Geometry check sheet. Reference: the model listing, model coordinates, mm. Coordinates: 2 decimals unless noted, no trailing zeros. Order: outer loops, then holes, each group sorted by start corner. A loop starts at its lowest first (then second) coordinate and runs counter-clockwise, first axis right, second up. Notation, with made-up numbers: (-34.5, -19) -> (6.5, -19) arc R11 cw to (6.5, -6) -> close; hole circle Ø5 at (42, -21). An arc over 180 degrees is marked (long way). Answer in a Markdown table with one row per item. Add a question column.
```python
from build123d import *

# Parameters (mm, degrees)
SKETCH_1_W          = 30
SKETCH_1_H          = 26.5
EXTRUDE_1_DEPTH     = 3
SKETCH_2_R          = 5
CUT_EXTRUDE_1_DEPTH = 30.15187029
SKETCH_3_R          = 2
CUT_EXTRUDE_2_DEPTH = 30.15187029
EXTRUDE_3_DEPTH     = 3
SKETCH_7_R          = 4
SKETCH_7_R_2        = 1.6
CUT_EXTRUDE_3_DEPTH = 3
FILLET_1_R          = 2
FILLET_2_R          = 2


with BuildPart() as part:
    # 草图1 → 凸台-拉伸1 (new body)
    with BuildSketch(Plane(origin=(0, 0, 0), x_dir=(1, 0, 0), z_dir=(0, 1, 0))):
        with Locations((-10.540723982, -0.479638009)):
            Rectangle(SKETCH_1_W, SKETCH_1_H)
    extrude(amount=EXTRUDE_1_DEPTH)

    # 草图2 → 切除-拉伸1 (cut, through all)
    with BuildSketch(Plane(origin=(0, 3, 0), x_dir=(1, 0, 0), z_dir=(0, 1, 0))):
        with Locations(Location((-10.540723982, -0.479638009, 0), (0, 0, 270))):
            Circle(SKETCH_2_R)
    extrude(amount=-CUT_EXTRUDE_1_DEPTH, mode=Mode.SUBTRACT)

    # 草图3 → 切除-拉伸2 (cut, through all)
    with BuildSketch(Plane(origin=(0, 3, 0), x_dir=(1, 0, 0), z_dir=(0, 1, 0))):
        with Locations(Location((-3.540723982, 7.520361991, 0), (0, 0, 270))):
            Circle(SKETCH_3_R)
        with Locations(Location((-17.540723982, 7.520361991, 0), (0, 0, 270))):
            Circle(SKETCH_3_R)
        with Locations(Location((-3.540723982, -8.479638009, 0), (0, 0, 270))):
            Circle(SKETCH_3_R)
        with Locations(Location((-17.540723982, -8.479638009, 0), (0, 0, 270))):
            Circle(SKETCH_3_R)
    extrude(amount=-CUT_EXTRUDE_2_DEPTH, mode=Mode.SUBTRACT)

    # 草图6 → 凸台-拉伸3 (add)
    with BuildSketch(Plane(origin=(4.459276018, 0, 0), x_dir=(0, 0, -1), z_dir=(1, 0, 0))):
        with BuildLine():
            Line((12.770361991, 3), (-13.729638009, 3))
            Line((-13.729638009, 3), (-13.729638009, -16.75))
            ThreePointArc((-13.729638009, -16.75), (-0.479638009, -30), (12.770361991, -16.75))
            Line((12.770361991, -16.75), (12.770361991, 3))
        make_face()
    extrude(amount=EXTRUDE_3_DEPTH)

    # 草图7 → 切除-拉伸3 (cut)
    with BuildSketch(Plane.ZY.offset(-4.459276018)):
        with Locations((0.479638009, -16.75)):
            Circle(SKETCH_7_R)
        with Locations((9.432771386, -16.75)):
            Circle(SKETCH_7_R_2)
        with Locations((-7.567228614, -16.75)):
            Circle(SKETCH_7_R_2)
    extrude(amount=-CUT_EXTRUDE_3_DEPTH, mode=Mode.SUBTRACT)

    # 圆角1
    fillet_1_edges = [part.edges().sort_by_distance(p)[0] for p in [
        (-25.540723982, 1.5, -12.770361991),
        (-25.540723982, 1.5, 13.729638009),
    ]]
    fillet(fillet_1_edges, radius=FILLET_1_R)

    # 圆角2
    fillet_2_edges = [part.edges().sort_by_distance(p)[0] for p in [
        (7.459276018, 3, 0.479638009),
        (4.459276018, 0, 0.479638009),
    ]]
    fillet(fillet_2_edges, radius=FILLET_2_R)


solid = part.part
```
(1) Cross-section at C-C (y = -13.5). Enter the section's corners in (x, z).
(2) Cross-section at A-A (x = 5). Enter the section's corners in (y, z).
(3) Cross-section at D-D (z = -7.5). Enter the section's corners in (x, y).
(4) Go/stop test with flat-tipped pins: P1, Ø10, axis at x = 1, z = 6, coming from the -Y side; P2, Ø12, axis at y = -7, z = 3, coming from the -X side; P3, Ø1, axis at y = -12.5, z = -1, coming from the -X side. Record where each tip stops, or that it passes through.
(5) Scan lines: line 1 along Z through (x, y) = (6, -16); line 2 along Y through (x, z) = (-15.5, -5); line 3 along X through (y, z) = (-26, 4.25). Record each from-to range of solid material in increasing order.
(6) Cross-section at B-B (z = 2.25). Enter the section's corners in (x, y).
(7) Mould release check, pull along X, two halves, no side actions. Record for faces 1 (the face through (-15, 0, -3)), 2 (the face through (-15.558, 1.521, 8.219)), 3 (the face through (7.459, -11, 1)): +X half, -X half, draft (parallel to the pull), parting line (faces both ways), or undercut.
Checks:
| question | item | result |
|---|---|---|
| 1 | outline | (4.46, -12.77) -> (7.46, -12.77) -> (7.46, -1.85) -> (4.46, -1.85) -> close; (4.46, 2.81) -> (7.46, 2.81) -> (7.46, 13.73) -> (4.46, 13.73) -> close |
| 2 | outline | (-16.75, -12.77) -> (3, -12.77) -> (3, 13.73) -> (-16.75, 13.73) arc R13.25 ccw to start; hole circle Ø8 at (-16.75, 0.48); hole circle Ø3.2 at (-16.75, -7.57); hole circle Ø3.2 at (-16.75, 9.43) |
| 3 | outline | (-25.54, 0) -> (-19.54, 0) -> (-19.54, 3) -> (-25.54, 3) -> close; (-15.54, 0) -> (-5.54, 0) -> (-5.54, 3) -> (-15.54, 3) -> close; (-1.54, 0) -> (2.46, 0) arc R2 cw to (4.46, -2) -> (4.46, -15.15) -> (7.46, -15.15) -> (7.46, 1) arc R2 ccw to (5.46, 3) -> (-1.54, 3) -> close; (4.46, -27.33) -> (7.46, -27.33) -> (7.46, -18.35) -> (4.46, -18.35) -> close |
| 4 | P1 | y = -29.86 |
| 4 | P2 | x = 4.19 |
| 4 | P3 | x = 4.46 |
| 5 | line 1 | -12.77 to -8.98, -6.15 to -3.45, 4.41 to 8.02, 10.85 to 13.73 |
| 5 | line 2 | 0 to 3 |
| 5 | line 3 | 4.46 to 7.46 |
| 6 | outline | (-25.54, 0) -> (-15.22, 0) -> (-15.22, 3) -> (-25.54, 3) -> close; (-5.86, 0) -> (2.46, 0) arc R2 cw to (4.46, -2) -> (4.46, -13.16) -> (7.46, -13.16) -> (7.46, 1) arc R2 ccw to (5.46, 3) -> (-5.86, 3) -> close; (4.46, -29.88) -> (7.46, -29.88) -> (7.46, -20.34) -> (4.46, -20.34) -> close |
| 7 | face 1 | draft |
| 7 | face 2 | undercut |
| 7 | face 3 | +X half |
